Input: part model. Units: mm. Frame: model coordinates. A direction names the side the tool comes from. Coordinates: 2 decimals unless noted, no trailing zeros. Order: outer loops, then holes, each group sorted by start corner. A loop starts at its lowest first (then second) coordinate and runs counter-clockwise, first axis right, second up. Notation, with made-up numbers: (32.5, 3) - (89.5, 3) arc R21 ccw to (89.5, 11) - close; hole circle Ø8 at (22.25, 45.25). An arc over 180 degrees is marked (long way). One line per question, with ' | ' between items. Start each with the question number.
```python
from build123d import *

# Parameters (mm, degrees)
F0_W      = 92.3617742956
F0_H      = 73.5575780272
F1_DEPTH  = 25.4
F2_DEPTH  = 25
F3_T      = -2.5
F3_FACE_W = 87.3617742956
F3_FACE_H = 68.5575780272


with BuildPart() as f1:
    # F0 (on Top) → F1 (new body)
    with BuildSketch(Plane.XY):
        with Locations((1.8435474485, 4.9775801599)):
            Rectangle(F0_W, F0_H)
    extrude(amount=F1_DEPTH)

    # F0 (on Top) → F2 (join)
    with BuildSketch(Plane.XY):
        with Locations((1.8435474485, 4.9775801599)):
            Rectangle(F0_W, F0_H)
    extrude(amount=F2_DEPTH)

    # F3
    f3_openings = [f1.faces().sort_by_distance(p)[0] for p in [
        (1.843547, 4.97758, 25.4),
    ]]
    offset(amount=F3_T, openings=f3_openings)

    # F3_face (on face) → F4 section 0
    with BuildSketch(Plane(origin=(1.8435474485, 4.9775801599, 2.5), x_dir=(1, 0, 0), z_dir=(0, 0, 1)), mode=Mode.PRIVATE) as f4_s0:
        Rectangle(F3_FACE_W, F3_FACE_H)
    loft([f4_s0.sketch, Vertex(0, 0, 0)])


solid = f1.part
```
(1) Reachability of faces 4 (the face through (1, 5, 0)), 5 (the face through (1, -29.301, 14)) from +Z, -Z, +X, -X, +Y, -Y: full face, straight path, thin tool, end or side. Return the list, or none.
(2) Material intervals for line 1 along X through (y, z) = (15, 11); line 2 along Y through (x, z) = (-1.5, 5.75); line 3 along Z through (x, y) = (21.5, 17.5), sorted ascending. Write a range as from..to.
(3) Section A-A (z = 23). Output: boundary loops of the cut face in (x, y), then the cut area to 3 significant figures.
(4) Pin query (flat end, axial travel): pin 1 (20.5 mm diameter, centred on x = -3.5, y = -5.5, fed in from +Z). Return the tip coordinate at first contact, or that it passes through.
(5) Section C-C (y = -13.5). Output: boundary loops of the cut face in (x, z).
(6) Draft query along X for faces 1 (the face through (-44.337, 4, 13)), 2 (the face through (1, 41.756, 13)), 3 (the face through (1, 39.256, 14)). Return one class per face: +X half, -X half, draft (parallel to the pull), parting line (faces both ways), or undercut.
(7) Section B-B (x = 7.5). Output: boundary loops of the cut face in (y, z), then the cut area to 3 significant figures.
Worked answers:
1) face 4: -Z, +X, -X, +Y, -Y | face 5: +Z
2) line 1: x = -44.34..-41.84, 45.52..48.02 | line 2: y = -31.8..-29.3, 39.26..41.76 | line 3: z = 0..2.5
3) outline: (-44.34, -31.8) - (48.02, -31.8) - (48.02, 41.76) - (-44.34, 41.76) - close; hole (-41.84, -29.3) - (45.52, -29.3) - (45.52, 39.26) - (-41.84, 39.26) - close | area: 805 mm²
4) pin 1: stops at z = 2.5
5) outline: (-44.34, 0) - (48.02, 0) - (48.02, 25.4) - (45.52, 25.4) - (45.52, 2.5) - (-41.84, 2.5) - (-41.84, 25.4) - (-44.34, 25.4) - close
6) face 1: -X half | face 2: draft | face 3: undercut
7) outline: (-31.8, 0) - (41.76, 0) - (41.76, 25.4) - (39.26, 25.4) - (39.26, 2.5) - (-29.3, 2.5) - (-29.3, 25.4) - (-31.8, 25.4) - close | area: 298 mm²
